The listing builds one solid part. Answer for the finished solid, in the listing's coordinates (mm). Face numbers are marked on the shaded views. A direction names the side the tool comes from. Coordinates: 2 decimals unless noted, no trailing zeros. Loops run counter-clockwise (first coordinate to the right, second up) from the corner with the lowest first, then second, coordinate; pieces in that order, holes last. Notation, with made-up numbers: M 86.5,16.5 L 132.5,16.5 A13 cw 132.5,28.5 Z; hole C 11.5,-23 d4. An arc over 180 degrees is marked long. Answer in a Markdown table with one row per item. Add a question column.
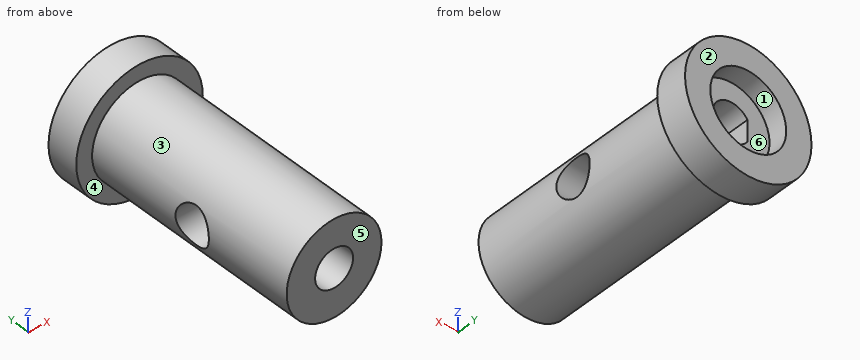
from build123d import *

# Parameters (mm, degrees)
SKETCH1_R                   = 10
METALSTOCK_DEPTH            = 40
EXTERIORLATHE_START         = -5
SKETCH2_OUTSIDE_W           = 31.798
SKETCH2_OUTSIDE_H           = 31.798
SKETCH2_OUTSIDE_R           = 7.5
EXTERIORLATHE_DEPTH         = 35
SKETCH6_R                   = 3
SHAFTHOLE_FOR_GEARBOX_DEPTH = 41
SKETCH7_W                   = 2
SKETCH7_H                   = 6
KEY_FOR_GEARBOX_DEPTH       = 12
SKETCH8_R                   = 3
SIDESCREWHOLE_DEPTH         = 11
SIDESCREWHOLE_DEPTH_BACK    = 11
SKETCH9_R                   = 6
GEARBOXCOUNTERSINK_DEPTH    = 3


with BuildPart() as part:
    # Sketch1 → MetalStock (new body)
    with BuildSketch(Plane(origin=(0, 0, 0), x_dir=(1, 0, 0), z_dir=(0, 1, 0))):
        Circle(SKETCH1_R)
    extrude(amount=-METALSTOCK_DEPTH)

    # Sketch2 outside → ExteriorLathe (cut)
    with BuildSketch(Plane(origin=(0, 0, 0), x_dir=(1, 0, 0), z_dir=(0, 1, 0)).offset(EXTERIORLATHE_START)):
        Rectangle(SKETCH2_OUTSIDE_W, SKETCH2_OUTSIDE_H)
        Circle(SKETCH2_OUTSIDE_R, mode=Mode.SUBTRACT)
    extrude(amount=-EXTERIORLATHE_DEPTH, mode=Mode.SUBTRACT)

    # Sketch6 → ShaftHole for Gearbox (cut, through all)
    with BuildSketch(Plane(origin=(0, 0, 0), x_dir=(1, 0, 0), z_dir=(0, 1, 0))):
        Circle(SKETCH6_R)
    extrude(amount=-SHAFTHOLE_FOR_GEARBOX_DEPTH, mode=Mode.SUBTRACT)

    # Sketch7 → Key for Gearbox (add)
    with BuildSketch(Plane(origin=(0, 0, 0), x_dir=(1, 0, 0), z_dir=(0, 1, 0))):
        with Locations((-3.5, 0)):
            Rectangle(SKETCH7_W, SKETCH7_H)
    extrude(amount=-KEY_FOR_GEARBOX_DEPTH)

    # Sketch8 → SideScrewHole (cut, two sides)
    with BuildSketch(Plane(origin=(0, 0, 0), x_dir=(0, 0, -1), z_dir=(1, 0, 0))) as sidescrewhole_sk:
        with Locations((0, -23)):
            Circle(SKETCH8_R)
    extrude(amount=SIDESCREWHOLE_DEPTH, mode=Mode.SUBTRACT)
    extrude(sidescrewhole_sk.sketch, amount=-SIDESCREWHOLE_DEPTH_BACK, mode=Mode.SUBTRACT)

    # Sketch9 → GearboxCounterSink (cut)
    with BuildSketch(Plane(origin=(0, 0, 0), x_dir=(1, 0, 0), z_dir=(0, 1, 0))):
        Circle(SKETCH9_R)
    extrude(amount=-GEARBOXCOUNTERSINK_DEPTH, mode=Mode.SUBTRACT)


solid = part.part
(1) A cutting plane is placed at A-A (z = 0). Give the vertices of the cut face in (x, y).
(2) A cutting plane is placed at B-B (x = -2). Give the vertices of the cut face in (y, z).
(3) A cutting plane is placed at C-C (y = -9). Give the vertices of the cut face in (x, z).
(4) A cutting plane is placed at D-D (y = -24). Give the vertices of the cut face in (x, z), plus the area to 3 significant figures.
(5) The mould has two halves that part along Z. Classify the marked faces 1, 2 and 3: released by +Z, released by -Z, zero draft, split by the parting line, or undercut.
(6) Straight lines are drawn through the part: line 1 (Z direction, x = 0, y = -28.5); line 2 (Y direction, x = 4.5, z = 0). For each, find the intervals that lie inside material, in ascending order.
(7) Each of these flat-tipped pins is pushed along its axis until it touches: pin 1 (1.7 mm diameter, centred on y = -6.5, z = 0, fed in from +X); pin 2 (2 mm diameter, centred on y = -14.5, z = -3.5, fed in from +X); pin 3 (6 mm diameter, centred on x = 1.5, y = -14, fed in from +Z). Where does it stop, or does it pass through?
(8) For the marked faces 4, 5 and 6, determine the directions among +Z, -Z, +X, -X, +Y, -Y from which every point of the face is accessible in a straight line to the end or side of a thin tool.
Solved:
| question | item | result |
|---|---|---|
| 1 | outline | M -10,-5 L -7.5,-5 L -7.5,-20 L -3,-20 L -3,-12 L -2.5,-12 L -2.5,-3 L -6,-3 L -6,0 L -10,0 Z; M -7.5,-40 L -3,-40 L -3,-26 L -7.5,-26 Z; M 3,-40 L 7.5,-40 L 7.5,-26 L 3,-26 Z; M 3,-20 L 7.5,-20 L 7.5,-5 L 10,-5 L 10,0 L 6,0 L 6,-3 L 3,-3 Z |
| 2 | outline | M -40,-7.23 L -5,-7.23 L -5,-9.8 L 0,-9.8 L 0,-5.66 L -3,-5.66 L -3,-2.24 L -21,-2.24 A3 cw -25,-2.24 L -40,-2.24 Z; M -40,2.24 L -25,2.24 A3 cw -21,2.24 L -3,2.24 L -3,5.66 L 0,5.66 L 0,9.8 L -5,9.8 L -5,7.23 L -40,7.23 Z |
| 3 | outline | C 0,0 d15; hole M -2.5,-1.66 A3 ccw long -2.5,1.66 Z |
| 4 | outline | M -6.95,-2.83 A7.5 ccw 6.95,-2.83 L 1,-2.83 A3 cw -1,-2.83 Z; M -6.95,2.83 L -1,2.83 A3 cw 1,2.83 L 6.95,2.83 A7.5 ccw Z |
| 4 | area | 93.5 mm² |
| 5 | face 1 | undercut |
| 5 | face 2 | zero draft |
| 5 | face 3 | split by the parting line |
| 6 | line 1 | z = -7.5 to -3, 3 to 7.5 |
| 6 | line 2 | y = -40 to -26, -20 to -3 |
| 7 | pin 1 | stops at x = 7.5 |
| 7 | pin 2 | stops at x = 7.07 |
| 7 | pin 3 | stops at z = 7.5 |
| 8 | face 4 | -Y |
| 8 | face 5 | +Z, -Z, +X, -X, -Y |
| 8 | face 6 | +Y |
